For this review, take the finished solid that the model builds, in its own axes (mm). Face numbers are marked on the shaded views. A direction names the side the tool comes from. Round coordinates to 2 decimals unless told otherwise and drop trailing zeros. Order: outer loops, then holes, each group sorted by start corner. A loop starts at its lowest first (then second) coordinate and runs counter-clockwise, first axis right, second up. Notation, with made-up numbers: (25, -32) -> (37, -32) arc R32 cw to (37, -6) -> close; hole circle Ø5 at (-7, -6.75). An arc over 180 degrees is marked (long way). Answer in a Markdown table with one row per item.
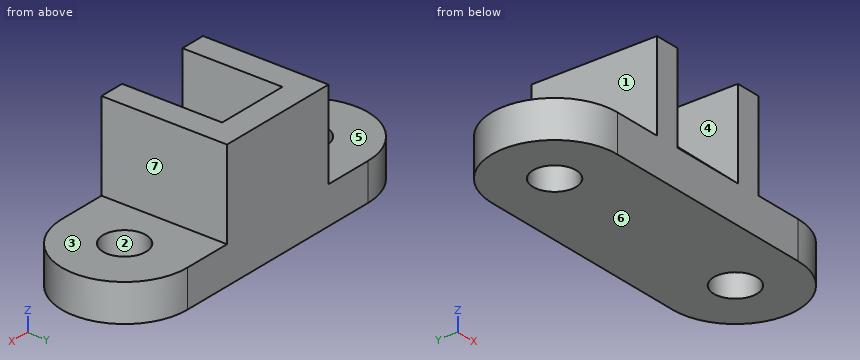
Autodesk Fusion 360 part; units mm, degrees
sketch "Sketch1" plane through (0, 0, 0) normal (0, 0, 1) x (1, 0, 0)
  line L0 (57, 32) -> (-57, 32)
  line L1 (-57, -32) -> (57, -32)
  circle A0 centre (57, 0) radius 11
  circle A1 centre (-57, 0) radius 11
  arc A2 (57, -32) -> (57, 32) centre (57, 0) ccw
  arc A3 (-57, 32) -> (-57, -32) centre (-57, 0) ccw
  line L2 (-57, -32) -> (-32, -32) construction
  line L3 (57, -32) -> (32, -32) construction
  dimension "d1" = 114
  dimension "d2" = 64
  dimension "d3" = 64
  dimension "d4" = 64
  dimension "d5" = 22
  dimension "d6" = 22
  dimension "d9" = 25
  dimension "d10" = 25
extrude "Extrude1" add sketch "Sketch1" along normal blind 19
sketch "Sketch2" plane through (0, 0, 0) normal (0, 1, 0) x (1, 0, 0)
  line L0 (-32, 0) -> (32, 0)
  line L1 (32, 0) -> (32, -64)
  line L2 (32, -64) -> (-32, -64)
  line L3 (-32, -64) -> (-32, 0)
  dimension "d11" = 64
extrude "Extrude2" add sketch "Sketch2" along normal mid plane 64
sketch "Sketch3" plane through (0, 0, 64) normal (0, 0, 1) x (-1, 0, 0)
  line L0 (-32, 32) -> (-32, -32)
  line L1 (-32, -32) -> (32, -32)
  line L2 (32, -32) -> (32, 32)
  line L3 (32, 32) -> (-32, 32)
  line L4 (32, 32) -> (32, -19)
  line L5 (-32, 32) -> (-32, -19)
  line L6 (32, 32) -> (19, 32)
  line L7 (-32, 32) -> (-19, 32)
  line L8 (19, 32) -> (19, -19)
  line L9 (-19, 32) -> (-19, -19)
  line L10 (-19, -19) -> (19, -19)
  dimension "d14" = 51
  dimension "d15" = 51
  dimension "d16" = 13
  dimension "d17" = 13
extrude "Extrude3" cut sketch "Sketch3" against normal blind 45 contours L3 L8 L9 L10
sketch "Sketch4" plane through (19, 0, 0) normal (-1, 0, 0) x (0, -1, 0)
  line L0 (32, 64) -> (-19, 64)
  line L1 (-19, 64) -> (-19, 19)
  line L2 (-19, 19) -> (32, 19)
  line L3 (32, 19) -> (32, 64)
  line L4 (-19, 64) -> (32, 19)
extrude "Extrude4" add sketch "Sketch4" along normal blind 38 contours L1 L2 L4
Q1. Clearance check with flat-ended pins moving along their axes: pin 1 Ø8 at (y, z) = (7.5, 54.5) entering from +X; pin 2 Ø1.5 at (y, z) = (-10.5, 48.5) entering from -X; pin 3 Ø5 at (x, y) = (55.5, -20.5) entering from +Z. State where each tip first meets the part, or that it passes through.
Answer key:
| item | result |
|---|---|
| pin 1 | stops at x = 32 |
| pin 2 | stops at x = -32 |
| pin 3 | stops at z = 19 |
Q2. Take a section at B-B, the plane y = 0. Write out the cut boundary in (x, z), then the cut area to 3 significant figures.
Answer key:
| item | result |
|---|---|
| outline | (-89, 0) -> (-68, 0) -> (-68, 19) -> (-89, 19) -> close; (-46, 0) -> (46, 0) -> (46, 19) -> (32, 19) -> (32, 64) -> (19, 64) -> (19, 47.24) -> (-19, 47.24) -> (-19, 64) -> (-32, 64) -> (-32, 19) -> (-46, 19) -> close; (68, 0) -> (89, 0) -> (89, 19) -> (68, 19) -> close |
| area | 4,790 mm^2 |
Q3. To check wall thickness, follow probe 1 along Y at (x, z) = (-57, 9); probe 2 along X at (y, z) = (-25, 59); probe 3 along X at (y, z) = (21, 51.5). State the ranges of each line that lie inside material, in increasing order.
Answer key:
| item | result |
|---|---|
| probe 1 | y = -32 to -11, 11 to 32 |
| probe 2 | x = -32 to -19, 19 to 32 |
| probe 3 | x = -32 to 32 |
Q4. Take a section at C-C, the plane x = 17. Write out the cut boundary in (y, z), then the cut area to 3 significant figures.
Answer key:
| item | result |
|---|---|
| outline | (-32, 0) -> (32, 0) -> (32, 64) -> (19, 64) -> (-32, 19) -> close |
| area | 2,950 mm^2 |
Q5. Tool access review of the marked faces 4, 5, 6 and 7: name each direction out of +Z, -Z, +X, -X, +Y, -Y from which nothing blocks a thin tool from reaching the whole face with its end or side.
Answer key:
| item | result |
|---|---|
| face 4 | +Z, -Y |
| face 5 | +Z, -X, +Y, -Y |
| face 6 | -Z, +X, -X, +Y, -Y |
| face 7 | +Z, +X, +Y, -Y |
Q6. The part is to be moulded in two halves that separate along X. For the marked faces 1, 2 and 3, say which applies: +X half, -X half, draft (parallel to the pull), parting line (faces both ways), or undercut.
Answer key:
| item | result |
|---|---|
| face 1 | -X half |
| face 2 | undercut |
| face 3 | draft |
Q7. Take a section at D-D, the plane y = -17. Write out the cut boundary in (x, z).
Answer key:
| item | result |
|---|---|
| outline | (-84.11, 0) -> (84.11, 0) -> (84.11, 19) -> (32, 19) -> (32, 64) -> (19, 64) -> (19, 32.24) -> (-19, 32.24) -> (-19, 64) -> (-32, 64) -> (-32, 19) -> (-84.11, 19) -> close |
Q8. Take a section at A-A, the plane z = 50.5. Write out the cut boundary in (x, y).
Answer key:
| item | result |
|---|---|
| outline | (-32, -32) -> (-19, -32) -> (-19, 3.7) -> (19, 3.7) -> (19, -32) -> (32, -32) -> (32, 32) -> (-32, 32) -> close |
